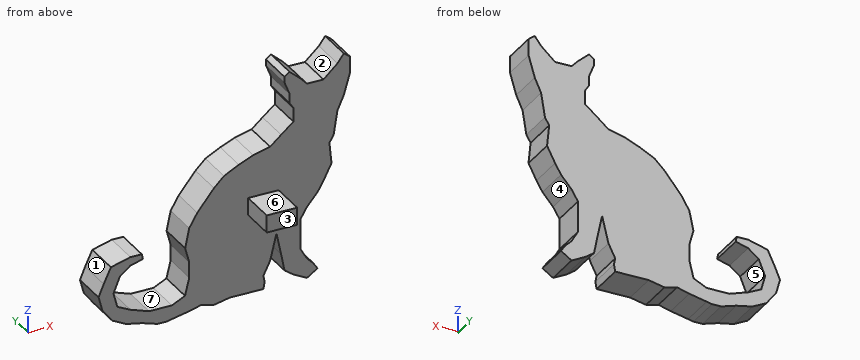
from build123d import *

# Parameters (mm, degrees)
F1_DEPTH = 12.7
F2_W     = 10.860083
F2_H     = 6.205762
F3_DEPTH = 12.7


with BuildPart() as f1:
    # F0 (on Front) → F1 (new body)
    with BuildSketch(Plane.XZ):
        Polygon((10.930421, 22.717176), (4.900595, 21.209723), (-0.224752, 19.099282), (-5.500847, 16.385859), (-9.036702, 12.918709), (-14.997827, 5.532174), (-17.861986, 0.708314), (-19.316724, -6.225982), (-17.861986, -11.652825), (-17.861986, -17.230413), (-19.369447, -23.410983), (-24.038606, -25.672167), (-32.182822, -25.672167), (-38.807783, -23.410983), (-43.465309, -21.149799), (-44.845456, -16.001211), (-42.584272, -10.446859), (-38.807783, -7.418466), (-34.359269, -6.225982), (-34.745501, -4.365046), (-38.807783, -4.365046), (-45.749934, -6.225982), (-48.312606, -11.652825), (-50.144989, -16.001211), (-48.764841, -21.149799), (-45.297699, -25.672167), (-40.323088, -28.184597), (-34.594753, -29.356468), (-29.167914, -31.04079), (-25.977362, -31.04079), (-24.038606, -30.638407), (-17.861986, -29.356468), (-13.490366, -28.184597), (-9.036702, -29.356468), (-3.390411, -28.184597), (1.584193, -28.184597), (8.518493, -28.184597), (8.987795, -25.672167), (8.518493, -23.410983), (10.930421, -18.587123), (13.191605, -9.240893), (14.849806, -17.230413), (16.055772, -23.410983), (19.221431, -25.672167), (24.045291, -28.184597), (27.813932, -25.672167), (26.306475, -23.410983), (24.045291, -21.149799), (21.784107, -17.230413), (21.784107, -12.105062), (21.784107, -6.225982), (24.045291, -2.457341), (27.813932, 1.91428), (29.924371, 5.532174), (32.788538, 11.109764), (32.034809, 18.647043), (33.542265, 21.209723), (34.898975, 29.651476), (37.16016, 34.62608), (39.371106, 42.163363), (39.371106, 48.042437), (37.16016, 49.700646), (34.898975, 46.685731), (29.924371, 42.163363), (27.813932, 42.163363), (24.045291, 42.163363), (21.784107, 44.575287), (17.864721, 48.042437), (16.055772, 46.685731), (16.055772, 44.575287), (17.864721, 40.052927), (17.864721, 36.736517), (19.221431, 34.62608), (19.221431, 29.651476), (14.849806, 26.033579), align=None)
    extrude(amount=F1_DEPTH)

    # F2 (on face) → F3 (join)
    with BuildSketch(Plane.XZ.offset(12.7)):
        with Locations((8.532922, 3.102881)):
            Rectangle(F2_W, F2_H)
    extrude(amount=F3_DEPTH)


solid = f1.part
Build history of the part. All positions in model axes, mm. Face numbers are marked on the shaded views. A direction names the side the tool comes from. Give positions to 0.01 mm unless a question says otherwise; leave off trailing zeros. Order: outer loops, then holes, each group sorted by start corner. A loop starts at its lowest first (then second) coordinate and runs counter-clockwise, first axis right, second up. Notation, with made-up numbers: M 12,51 L 61,51 A22 ccw 61,77 Z; hole C -18,45 d11. An arc over 180 degrees is marked long. Use one line per item in the form item = value.
Q1. Pin check, flat tips, straight feed: P1, Ø9.5, axis at x = 3, y = -8.5, coming from the -Z side; P2, Ø3, axis at x = -1, y = -12, coming from the +Z side; P3, Ø4.5, axis at x = -37, y = -8.5, coming from the +Z side. Stop position of each tip, or through.
Conclusion:
P1 = -28.18
P2 = 19.4
P3 = -4.37
Q2. Slice it at A-A, the plane z = -13. Write the cut outline in (x, y), and give its area (3 significant figures).
Conclusion:
outline = M -48.88,-12.7 L -43.62,-12.7 L -43.62,0 L -48.88,0 Z; M -17.86,-12.7 L 12.28,-12.7 L 12.28,0 L -17.86,0 Z; M 13.97,-12.7 L 21.78,-12.7 L 21.78,0 L 13.97,0 Z
area = 549 mm2
Q3. Slice it at C-C, the plane z = 14.5. Write the cut outline in (x, y).
Conclusion:
outline = M -7.42,-12.7 L 32.45,-12.7 L 32.45,0 L -7.42,0 Z
Q4. Wall check: probe 1 along X at (y, z) = (-2, -22); probe 2 along Y at (x, z) = (-15.5, -11); probe 3 along Z at (x, y) = (4.5, -22). Give the ranges that are in metal, low to high.
Conclusion:
probe_1 = -48.11 to -41.71, -19.03 to 9.22, 15.78 to 24.9
probe_2 = -12.7 to 0
probe_3 = 0 to 6.21
Q5. Pull direction X, two halves, no side cores. Call the marked faces 1, 2 and 3: released by +X, released by -X, zero draft, split by the parting line, or undercut.
Conclusion:
face_1 = released by -X
face_2 = undercut
face_3 = zero draft
Q6. Slice it at B-B, the plane y = -22.25. Write the cut outline in (x, z).
Conclusion:
outline = M 3.1,0 L 13.96,0 L 13.96,6.21 L 3.1,6.21 Z
Q7. Which spindle directions (+Z, -Z, +X, -X, +Y, -Y) get a long thin tool onto all of the face, cutting with end or side? Do the marked faces 4, 5, 6 and 7. Say none if no direction does.
Conclusion:
face_4 = +X, +Y, -Y
face_5 = +Y, -Y
face_6 = +Z, +X, -X, -Y
face_7 = +Z, +Y, -Y
